The listing builds one solid part. Answer for the finished solid, in the listing's coordinates (mm). A direction names the side the tool comes from. Give positions to 0.01 mm unless a question says otherwise; leave off trailing zeros. Order: outer loops, then holes, each group sorted by start corner. A loop starts at its lowest first (then second) coordinate and runs counter-clockwise, first axis right, second up. Notation, with made-up numbers: (22.25, -3.75) - (58.25, -3.75) arc R17 ccw to (58.25, 22.25) - close; hole circle Ø8 at (-8.5, 64.25). An arc over 180 degrees is marked (long way). Answer as CSV lines item,"result". Start each with the question number.
1. Section A-A on x = 9.5 is taken. Give the vertices of the cut face in (y, z), and give its area (3 significant figures).
2. Flat-ended cylindrical pins translate along their axes: pin 1 (1 mm diameter, centred on x = -12.5, y = 1, fed in from -Z); pin 2 (2 mm diameter, centred on x = 6, z = 3, fed in from -Y); pin 3 (1 mm diameter, centred on x = -3, z = -1, fed in from -Y). Find the tip coordinate at first contact, or state that the pin passes through.
3. Which of the six approach directions +Z, -Z, +X, -X, +Y, -Y give full straight-line access (tool end or side, diameter ignored) to faces 1 (the flat face through (-16, 0, 0)), 2 (the cylindrical face through (10.01, -1.978, -2.579))?
4. Section B-B on x = -3 is taken. Give the vertices of the cut face in (y, z).
5. Consider line 1 along X through (y, z) = (2.25, 0.5); line 2 along Z through (x, y) = (10, 0); line 3 along Y through (x, z) = (10, -1.75). Determine where each line is inside the solid, lowest interval first. Write a range as [from, to].
6. Determine the mould class of faces 3 (the flat face through (16, 0, 0)), 4 (the cylindrical face through (0.08, 2.23, 0.29)), 5 (the cylindrical face through (-10.01, -1.978, -2.579)), 6 (the cylindrical face through (-15.254, 0.165, -3.746)) for opening direction X: +X half, -X half, draft (parallel to the pull), parting line (faces both ways), or undercut.
from build123d import *

# Parameters (mm, degrees)
SKETCH1_R            = 2.25
BOSS_EXTRUDE1_DEPTH  = 6
SKETCH2_R            = 3.25
BOSS_EXTRUDE2_DEPTH  = 10
SKETCH3_R            = 3.75
BOSS_EXTRUDE3_DEPTH  = 1.5
FILLET1_R            = 0.5
FILLET2_R            = 0.5
FILLET1_OF_MIRROR1_R = 0.5
FILLET2_OF_MIRROR1_R = 0.5


with BuildPart() as part:
    # Sketch1 → Boss-Extrude1 (new, symmetric)
    with BuildSketch(Plane(origin=(0, 0, 0), x_dir=(0, 0, -1), z_dir=(1, 0, 0))):
        Circle(SKETCH1_R)
    extrude(amount=BOSS_EXTRUDE1_DEPTH, both=True)

    # Sketch2 → Boss-Extrude2 (add)
    with BuildSketch(Plane.ZY.offset(6)):
        Circle(SKETCH2_R)
    boss_extrude2 = extrude(amount=BOSS_EXTRUDE2_DEPTH)

    # Sketch3 → Boss-Extrude3 (add)
    with BuildSketch(Plane.ZY.offset(16)):
        Circle(SKETCH3_R)
    boss_extrude3 = extrude(amount=-BOSS_EXTRUDE3_DEPTH)

    # Fillet1
    fillet1_edges = [part.edges().sort_by_distance(p)[0] for p in [
        (-14.5, 0, -3.75),
        (-16, 0, -3.75),
    ]]
    fillet(fillet1_edges, radius=FILLET1_R - 0.0001)  # a hair under: the kernel refuses the full size

    # Fillet2
    fillet2_edges = [part.edges().sort_by_distance(p)[0] for p in [
        (-14.5, 0, -3.25),
    ]]
    fillet(fillet2_edges, radius=FILLET2_R)

    # Mirror1: Boss-Extrude2, Boss-Extrude3 across plane
    add(boss_extrude2.mirror(Plane(origin=(0, 0, 0), x_dir=(0, 0, 1), z_dir=(1, 0, 0))))
    add(boss_extrude3.mirror(Plane(origin=(0, 0, 0), x_dir=(0, 0, 1), z_dir=(1, 0, 0))))

    # Fillet1 of Mirror1
    fillet1_of_mirror1_edges = [part.edges().sort_by_distance(p)[0] for p in [
        (14.5, 0, -3.75),
        (16, 0, -3.75),
    ]]
    fillet(fillet1_of_mirror1_edges, radius=FILLET1_OF_MIRROR1_R - 0.0001)  # a hair under: the kernel refuses the full size

    # Fillet2 of Mirror1
    fillet2_of_mirror1_edges = [part.edges().sort_by_distance(p)[0] for p in [
        (14.5, 0, -3.25),
    ]]
    fillet(fillet2_of_mirror1_edges, radius=FILLET2_OF_MIRROR1_R)


solid = part.part
Checks:
1,outline,"circle Ø6.5 at (0, 0)"
1,area,"33.2 mm²"
2,pin 1,"stops at z = -3.21"
2,pin 2,"stops at y = -2.56"
2,pin 3,"stops at y = -2.19"
3,face 1,"+Z, -Z, -X, +Y, -Y"
3,face 2,"none"
4,outline,"circle Ø4.5 at (0, 0)"
5,line 1,"x = [-16, -6], [6, 16]"
5,line 2,"z = [-3.25, 3.25]"
5,line 3,"y = [-2.74, 2.74]"
6,face 3,"+X half"
6,face 4,"undercut"
6,face 5,"undercut"
6,face 6,"draft"
